Design review of the part built by this model. Coordinates are the model's own, in mm. Give positions to 0.01 mm unless a question says otherwise; leave off trailing zeros. Write each loop counter-clockwise with the first axis right and the second up, starting at its lowest first coordinate (ties: lowest second). Pieces come first, ordered by that corner, then holes. Notation, with made-up numbers: M -24.5,-6.75 L 24.5,-6.75 A27 ccw 24.5,27.25 Z; hole C 6,11.25 d6. An arc over 180 degrees is marked long. Use a Markdown table: item, result. Add a question column.
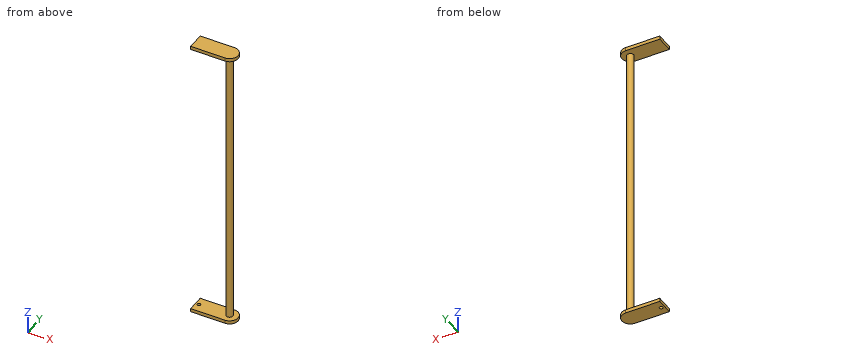
Autodesk Inventor part; units mm, degrees
ref_plane "YZ Plane" through (0, 0, 0) normal (1, 0, 0) x (0, 1, 0)
ref_plane "XZ Plane" through (0, 0, 0) normal (0, 1, 0) x (-1, 0, 0)
ref_plane "XY Plane" through (0, 0, 0) normal (0, 0, 1) x (1, 0, 0)
sketch "Skizze1" plane through (0, 0, 0) normal (0, 0, 1) x (1, 0, 0)
  circle A0 centre (0, 0) radius 9.75
  dimension "d0" = 19.5
extrude "Extrusion1" add sketch "Skizze1" along normal blind 830
sketch "Skizze4" plane through (0, 0, 830) normal (0, 0, 1) x (1, 0, 0)
  arc A0 (0, -25) -> (0, 25) centre (0, 0) ccw
  line L0 (0, 0) -> (0, -25) construction
  line L1 (0, 0) -> (0, 27.5151) construction
  line L2 (0, 25) -> (-100, 25)
  line L3 (-100, 25) -> (-100, -25)
  line L4 (-100, -25) -> (0, -25)
  point P0 (0, 25)
  dimension "d9" = 180
  dimension "d10" = 100
  dimension "d11" = 50
  dimension "d12" = 25
extrude "Extrusion4" add sketch "Skizze4" along normal blind 10
sketch "Skizze5" plane through (0, 0, 0) normal (0, 0, -1) x (-1, 0, 0)
  arc A0 (0, 25) -> (0, -25) centre (0, 0) ccw
  line L0 (0, 25) -> (100, 25)
  line L1 (100, 25) -> (100, -25)
  line L2 (100, -25) -> (0, -25)
  dimension "d15" = 25
  dimension "d16" = 0
  dimension "d17" = 0
  dimension "d18" = 100
  dimension "d19" = 50
  dimension "d20" = 90
extrude "Extrusion5" add sketch "Skizze5" along normal blind 10
sketch "Skizze6" plane through (0, 0, 0) normal (0, 0, 1) x (1, 0, 0)
  circle A0 centre (-90, 0) radius 5
  line L0 (-100, 25) -> (0, 25)
  line L1 (-100, -25) -> (-100, 25)
  point P0 (0, 0)
  dimension "d23" = 10
  dimension "d24" = 25
  dimension "d25" = 10
extrude "Extrusion6" cut sketch "Skizze6" against normal up to surface (10 mm away)
properties part number "LenkungHinten"
(1) For pin 1 (12 mm diameter, centred on y = 6, z = 163.5, fed in from -X); pin 2 (6 mm diameter, centred on x = -6.5, z = 146.5, fed in from +Y); pin 3 (5 mm diameter, centred on y = 5.5, z = 349, fed in from -X), all flat-tipped, find the tip position at first contact; note any pin that passes through.
(2) Add section A-A on x = -21.5. Give the boundary of the cut face in (y, z).
(3) Wall thickness on L1, parallel to Z at x = 20.5, y = 0.5; L2, parallel to Y at x = -90, z = -8; L3, parallel to Z at x = -88, y = 3.5: over which ranges is each line inside the solid? List them lowest first.
(4) Add section B-B on z = 152. Give the boundary of the cut face in (x, y).
From the geometry:
| question | item | result |
|---|---|---|
| 1 | pin 1 | stops at x = -9.75 |
| 1 | pin 2 | stops at y = 9.1 |
| 1 | pin 3 | stops at x = -9.28 |
| 2 | outline | M -25,-10 L 25,-10 L 25,0 L -25,0 Z; M -25,830 L 25,830 L 25,840 L -25,840 Z |
| 3 | L1 | z = -10 to 0, 830 to 840 |
| 3 | L2 | y = -25 to -5, 5 to 25 |
| 3 | L3 | z = 830 to 840 |
| 4 | outline | C 0,0 d19.5 |
